Autodesk Inventor part; units mm, degrees
ref_plane "Work Plane1" through (29, 0, 0) normal (0, -1, 0) x (1, 0, 0)
ref_plane "YZ Plane" through (0, 0, 0) normal (1, 0, 0) x (0, 1, 0)
ref_plane "XZ Plane" through (0, 0, 0) normal (0, 1, 0) x (-1, 0, 0)
sketch "Sketch1" plane through (0, 0, 0) normal (0, 0, 1) x (1, 0, 0)
  line L0 (-0.9667, 0) -> (35, 0)
  line L1 (35, 0) -> (35, 2.5)
  line L2 (35, 2.5) -> (19, 2.5)
  line L3 (19, 2.5) -> (18.5091, 2.5)
  line L4 (18.5091, 2.5) -> (0, 2.5)
  line L5 (0, 2.5) -> (0, 4.25)
  line L6 (0, 4.25) -> (-5, 4.25)
  line L7 (-5, 4.25) -> (-5, 2.3094)
  line L8 (-5, 2.3094) -> (-2.3, 2.3094)
  line L9 (-2.3, 2.3094) -> (-0.9667, 0)
  line L10 (-13, 0) -> (43, 0)
  line L11 (0, -0.85) -> (0, 5.1)
  line L12 (19, 2.5) -> (0, 2.5) construction
  dimension "d1" = 16
  dimension "d2" = 0.4909
  dimension "d3" = 5
  dimension "d4" = 2.7
  dimension "d5" = 60
  dimension "d6" = 5
  dimension "d7" = 5
  dimension "d8" = 4.6188
  dimension "d9" = 8.5
  dimension "d26" = 35
revolve "Body" add sketch "Sketch1" angle 360 about axis through (-0.9667, 0, 0) along (1, 0, 0)
sketch "Sketch2" plane through (-5, 0, 0) normal (-1, 0, 0) x (0, 0, 1)
  circle A0 centre (0, 0) radius 2.3094
  line L0 (0, -5.95) -> (0, 5.95)
  line L1 (-5.95, 0) -> (5.95, 0)
  line L2 (2.3094, 0) -> (1.1547, -2)
  line L3 (1.1547, -2) -> (-1.1547, -2)
  line L4 (-1.1547, -2) -> (-2.3094, 0)
  line L5 (-2.3094, 0) -> (-1.1547, 2)
  line L6 (-1.1547, 2) -> (1.1547, 2)
  line L7 (1.1547, 2) -> (2.3094, 0)
extrude "Slot" add sketch "Sketch2" against normal up to next contours L7 A0 | A0 L2 | L6 L0 A0 | A0 L0 L3 | L0 L6 A0 | A0 L3 L0 | L4 A0 | A0 L5
fillet "Fillet1" radius 0.4 1 edges at (-5, -4.25, 0)
thread "Thread"
chamfer "Chamfer1" distance 0.4908 distance2 0.4908 1 edges at (35, -2.5, 0) measured on face at (35, -0.7192, 0.1653)
ref_plane "Work Plane1" through (29, 0, 0) normal (0, -1, 0) x (1, 0, 0)
fillet "Fillet2" radius 0.1 1 edges at (0, -2.5, 0)
equation "\"d30\" = R"
equation "\"d17\" = RR"
equation "\"d13\" = GEL"
equation "\"d15\" = -0.5 * SPD + 0.5 * GD"
equation "\"d16\" = GUL"
equation "\"d1\" = GEL"
equation "\"d3\" = KOH"
equation "\"d4\" = INTI"
equation "\"d6\" = GD"
equation "\"d7\" = BDM"
equation "\"d8\" = 1.1547 * SW"
equation "\"d9\" = KOD"
equation "\"d26\" = NLG"
equation "\"GD\" = NND"
equation "\"NLG\" = 35"
equation "\"GEL\" = 16"
equation "\"KOD\" = 8.5"
equation "\"KOH\" = NND"
equation "\"INTI\" = 2.7"
equation "\"GAL\" = 0.61345 * PTC"
equation "\"GUL\" = 0.61345 * PTC"
equation "\"BDM\" = NND"
equation "\"SW\" = 4"
equation "\"RR\" = 0.4"
equation "\"SPD\" = NND - 1.2269 * PTC"
equation "\"R\" = 0.1"
equation "\"TOA\" = 30deg"
equation "\"GD1\" = THREADDIA - 1.2269 * PTC"
equation "\"THREADDIA\" = 5"
equation "\"FAWI\" = 45deg"
equation "\"PTC\" = 0.8"
equation "\"NND\" = 5"
equation "\"E0\" = 1.155 * SW"
equation "\"PHH\" = 0"
properties part number "CSN 02 1143 - M5 x 35" material "Steel, Mild"
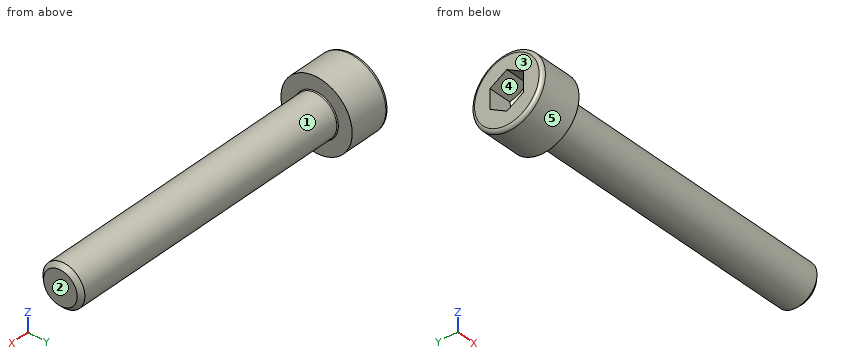
CAD build for the part. Positions are in the model's coordinates, mm. Face numbers are marked on the shaded views. A direction names the side the tool comes from. Coordinates: 2 decimals unless noted, no trailing zeros. Write each loop counter-clockwise with the first axis right and the second up, starting at its lowest first coordinate (ties: lowest second). Pieces come first, ordered by that corner, then holes. Notation, with made-up numbers: (35.25, 0.25) -> (67.25, 0.25) arc R24 ccw to (67.25, 24.25) -> close; hole circle Ø2 at (-11.75, -22). An arc over 180 degrees is marked (long way). Use CSV: the item, a comma, the result in double quotes. Start each with the question number.
Item 1: Drop flat-ended pins along their axis: P1, Ø1, axis at x = 8.5, y = -1.5, coming from the -Z side; P2, Ø5, axis at x = 18.5, y = -1.5, coming from the -Z side. Give the stop position or say it passes through.
Item 2: Band-saw the part on A-A, the plane x = 31. Write the cut outline in (y, z).
Item 3: Two-plate mould, pull along Y, no slides. Class the marked faces 3, 4 and 5: +Y half, -Y half, draft (parallel to the pull), parting line (faces both ways), or undercut.
Item 4: Wall check: probe 1 along X at (y, z) = (2.75, -1); probe 2 along X at (y, z) = (1.75, 0); probe 3 along Y at (x, z) = (13, 1.5). Give the ranges that are in metal, low to high.
Item 5: Tool access for the marked faces 1 and 2: list every direction of +Z, -Z, +X, -X, +Y, -Y with a clear straight run to the whole face (end or side of a thin tool).
Response values:
1,P1,"stops at z = -2.29"
1,P2,"stops at z = -2.5"
2,outline,"circle Ø5 at (0, 0)"
3,face 3,"draft"
3,face 4,"undercut"
3,face 5,"parting line"
4,probe 1,"x = -5 to 0"
4,probe 2,"x = -1.98 to 35"
4,probe 3,"y = -2 to 2"
5,face 1,"+X"
5,face 2,"+Z, -Z, +X, +Y, -Y"
